Design review of the part shown in the three views and the two pictorial views. Dimensions are in mm from the part's minimum x, y and z. Round coordinates to 2 decimals unless told otherwise and drop trailing zeros. Loops run counter-clockwise (first coordinate to the right, second up) from the corner with the lowest first, then second, coordinate; pieces in that order, holes last. Notation, with made-up numbers: M -11,29.5 L 21,29.5 A37 ccw 21,68.5 Z; hole C 78,81 d1. An arc over 180 degrees is marked long. One line per question, with ' | ' between items. Start each with the question number.
1) For probe 1 along X at (y, z) = (15.25, 6.75); probe 2 along Y at (x, z) = (41, 5); probe 3 along Y at (x, z) = (25, 7.5), list the stretches that pass through material, from the lowest coordinate up. Write a range as from..to.
2) For pin 1 Ø5 at (x, y) = (25, 15) entering from +Z, flat-tipped, find the tip position at first contact; note if it passes through.
3) Mouldability with a two-part tool opening along X and no side actions: class the marked faces 1, 2 and 3 as pulls with the +X half, pulls with the -X half, needs draft (parallel to the pull), parting line crosses it, or undercut.
4) We need section A-A (y = 15). Give the boundary of the cut face in (x, z), and give its area (3 significant figures).
5) We need section B-B (x = 25). Give the boundary of the cut face in (y, z).
6) We need section D-D (x = 9). Give the boundary of the cut face in (y, z), and give its area (3 significant figures).
7) We need section C-C (z = 11). Give the boundary of the cut face in (x, y).
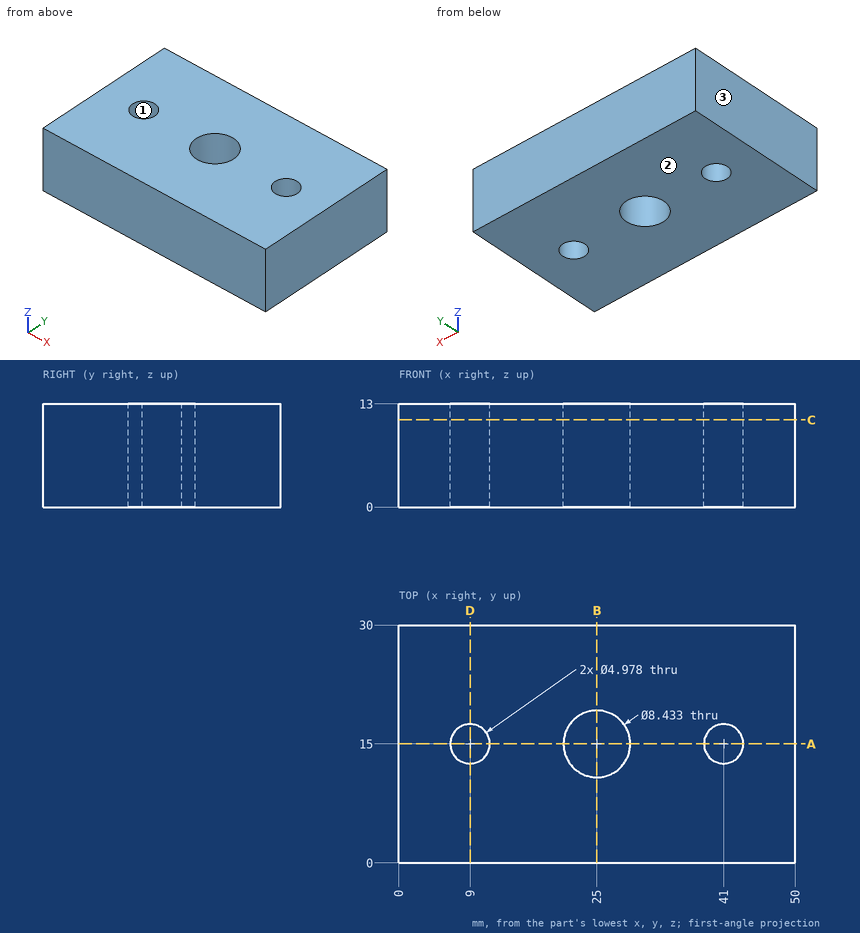
Answers below:
1) probe 1: 0..6.52, 11.48..20.79, 29.21..38.52, 43.48..50 | probe 2: 0..12.51, 17.49..30 | probe 3: 0..10.78, 19.22..30
2) pin 1: through
3) face 1: undercut | face 2: needs draft | face 3: pulls with the -X half
4) outline: M 0,0 L 6.51,0 L 6.51,13 L 0,13 Z; M 11.49,0 L 20.78,0 L 20.78,13 L 11.49,13 Z; M 29.22,0 L 38.51,0 L 38.51,13 L 29.22,13 Z; M 43.49,0 L 50,0 L 50,13 L 43.49,13 Z | area: 411 mm^2
5) outline: M 0,0 L 10.78,0 L 10.78,13 L 0,13 Z; M 19.22,0 L 30,0 L 30,13 L 19.22,13 Z
6) outline: M 0,0 L 12.51,0 L 12.51,13 L 0,13 Z; M 17.49,0 L 30,0 L 30,13 L 17.49,13 Z | area: 325 mm^2
7) outline: M 0,0 L 50,0 L 50,30 L 0,30 Z; hole C 9,15 d4.98; hole C 25,15 d8.43; hole C 41,15 d4.98
